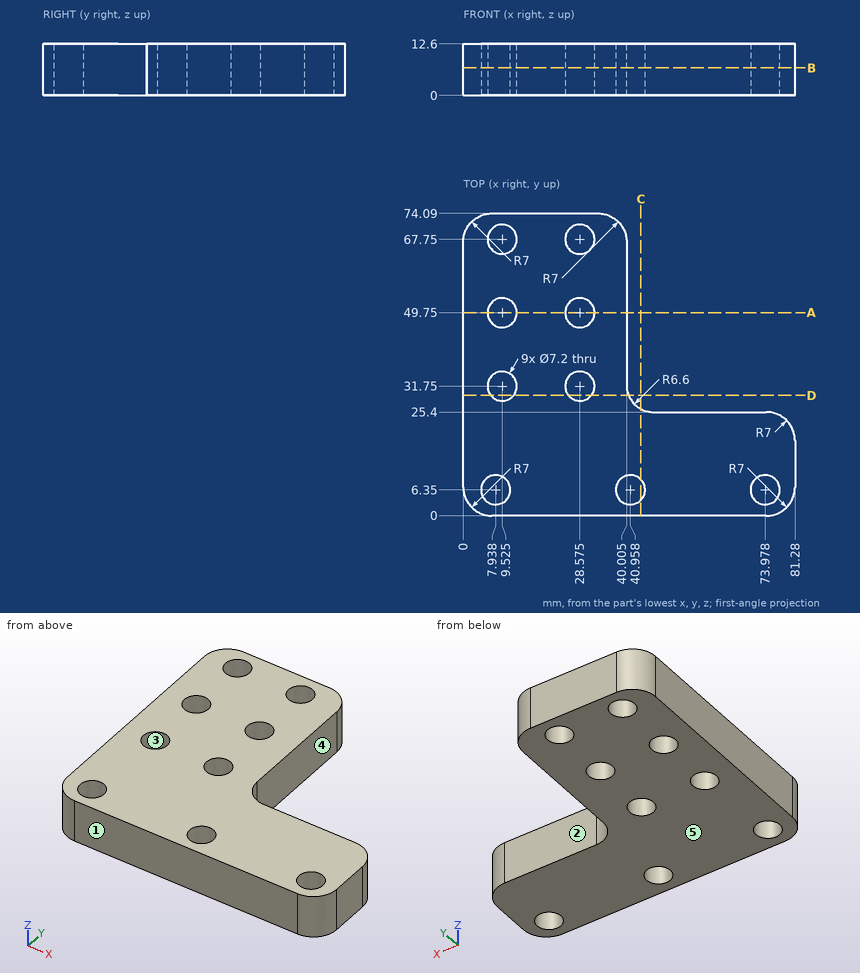
Answer from the drawing. Dimensions are ordinates in mm from the lowest x, y and z of the part. A direction names the side the tool comes from. Coordinates: 2 decimals unless noted, no trailing zeros. Write each loop counter-clockwise with the first axis right and the second up, starting at its lowest first coordinate (ties: lowest second). Pieces come first, ordered by that corner, then holes. Notation, with made-up numbers: M -20.5,76 L -16.5,76 A20 ccw -16.5,80 Z; hole C 13,-33 d2. An arc over 180 degrees is marked long. Use one line per item in the form item = value. Start each with the question number.
1. Each of these flat-tipped pins is pushed along its axis until it touches: P1, Ø5, axis at x = 38.5, z = 7.5, coming from the +Y side; P2, Ø4, axis at y = 57, z = 8, coming from the +X side (1 decimal). Where does it stop, or does it pass through?
2. Straight lines are drawn through the part: probe 1 along X at (y, z) = (35, 10.5) (1 decimal); probe 2 along X at (y, z) = (67, 2) (1 decimal); probe 3 along X at (y, z) = (36, 6) (1 decimal). For each, find the intervals that lie inside material, in ascending order. Write a range as from..to.
3. The mould has two halves that part along Y. Classify the marked faces 1, 2 and 3: released by +Y, released by -Y, zero draft, split by the parting line, or undercut.
4. A tool of negligible diameter and unlimited length cuts with its end or side. For the marked faces 4 and 5, from which of +Z, -Z, +X, -X, +Y, -Y can it reach the whole face along a straight path? Write none if from no direction.
5. The part is cut by section B-B (z = 6.75). Give the number of separate pieces and of enclosed holes in the cut face, plus the area to 3 significant figures.
6. The part is cut by section A-A (y = 49.75). Give the vertices of the cut face in (x, z) (1 decimal).
7. The part is cut by section C-C (x = 43.5). Give the vertices of the cut face in (y, z) (1 decimal).
8. The part is cut by section D-D (y = 29.5). Give the vertices of the cut face in (x, z) (1 decimal).
Evaluation:
q1.P1 = 73.42
q1.P2 = 40
q2.probe_1 = 0..8, 11.1..27, 30.1..40
q2.probe_2 = 0..6, 13..25.1, 32.1..40
q2.probe_3 = 0..40
q3.face_1 = released by -Y
q3.face_2 = released by +Y
q3.face_3 = undercut
q4.face_4 = +Z, -Z, +X, +Y
q4.face_5 = -Z, +X, -X, +Y, -Y
q5.separate_pieces = 1
q5.enclosed_holes = 9
q5.area = 3,600 mm^2
q6.outline = M 0,0 L 5.9,0 L 5.9,12.6 L 0,12.6 Z; M 13.1,0 L 25,0 L 25,12.6 L 13.1,12.6 Z; M 32.2,0 L 40,0 L 40,12.6 L 32.2,12.6 Z
q7.outline = M 0,0 L 3.8,0 L 3.8,12.6 L 0,12.6 Z; M 8.9,0 L 26.2,0 L 26.2,12.6 L 8.9,12.6 Z
q8.outline = M 0,0 L 6.7,0 L 6.7,12.6 L 0,12.6 Z; M 12.3,0 L 25.8,0 L 25.8,12.6 L 12.3,12.6 Z; M 31.4,0 L 40.5,0 L 40.5,12.6 L 31.4,12.6 Z
